from build123d import *

# Parameters (mm, degrees)
SKETCH1_R           = 100
SKETCH1_R_2         = 1.75
BOSS_EXTRUDE1_DEPTH = 2
BOSS_EXTRUDE2_DEPTH = 2


with BuildPart() as part:
    # Sketch1 → Boss-Extrude1 (new body)
    with BuildSketch(Plane.XY):
        Circle(SKETCH1_R)
        Circle(SKETCH1_R_2, mode=Mode.SUBTRACT)
    extrude(amount=BOSS_EXTRUDE1_DEPTH)

    # Sketch2 → Boss-Extrude2 (add)
    with BuildSketch(Plane.XY.offset(2)):
        Polygon((-1.25, -86), (1.25, -86), (3.25, -84), (-3.25, -84), align=None)
        Polygon((42.41156908, -80.578044827), (39.374382907, -74.271262752), (38.440212649, -76.940967966), (40.175747605, -80.544843437), align=None)
        Polygon((78.645827138, -58.561048264), (73.173006761, -54.196619651), (72.707858639, -56.383772418), (75.835184569, -58.877731625), align=None)
        Polygon((93.314928402, -22.58066955), (94.819742358, -24.975567242), (96.266128429, -18.638535813), (93.871230737, -20.14334977), align=None)
        Polygon((89.971519088, 19.253266034), (89.441633044, 17.080889275), (96.266128429, 18.638535813), (93.871230737, 20.14334977), align=None)
        Polygon((68.016869745, 52.642833607), (67.700186383, 49.832191038), (73.173006761, 54.196619651), (71.144195674, 55.136792814), align=None)
        Polygon((40.175747605, 80.544843437), (42.41156908, 80.578044827), (41.043515084, 82.346781173), align=None)
        Polygon((37.923325436, 81.629552785), (40.175747605, 80.544843437), (41.043515084, 82.346781173), (38.791092914, 83.431490521), align=None)
        Polygon((38.791092914, 83.431490521), (36.555271439, 83.398289131), (37.923325436, 81.629552785), align=None)
        Polygon((1.25, 86), (-1.25, 86), (-3.25, 84), (3.25, 84), align=None)
        Polygon((-42.41156908, 80.578044827), (-39.374382907, 74.271262752), (-38.440212649, 76.940967966), (-40.175747605, 80.544843437), align=None)
        Polygon((-78.645827138, 58.561048264), (-73.173006761, 54.196619651), (-72.707858639, 56.383772418), (-75.835184569, 58.877731625), align=None)
        Polygon((-93.314928402, 22.58066955), (-94.819742358, 24.975567242), (-96.266128429, 18.638535813), (-93.871230737, 20.14334977), align=None)
        Polygon((-89.971519088, -19.253266034), (-89.441633044, -17.080889275), (-96.266128429, -18.638535813), (-93.871230737, -20.14334977), align=None)
        Polygon((-68.016869745, -52.642833607), (-67.700186383, -49.832191038), (-73.173006761, -54.196619651), (-71.144195674, -55.136792814), align=None)
        Polygon((-40.175747605, -80.544843437), (-42.41156908, -80.578044827), (-41.043515084, -82.346781173), align=None)
        Polygon((-37.923325436, -81.629552785), (-40.175747605, -80.544843437), (-41.043515084, -82.346781173), (-38.791092914, -83.431490521), align=None)
        Polygon((-38.791092914, -83.431490521), (-36.555271439, -83.398289131), (-37.923325436, -81.629552785), align=None)
    extrude(amount=BOSS_EXTRUDE2_DEPTH)


solid = part.part
Can you work these out from the model? Positions are in its coordinate system, mm. A direction names the side the tool comes from. Coordinates: 2 decimals unless noted, no trailing zeros. Loops run counter-clockwise (first coordinate to the right, second up) from the corner with the lowest first, then second, coordinate; pieces in that order, holes last. Notation, with made-up numbers: M 46.25,86 L 91.25,86 A24 ccw 91.25,124 Z; hole C 51.25,68 d9. An arc over 180 degrees is marked long. Return JSON: item names as keys, results as strings. Group by question number.
Item 1: I'm going to push flat-ended pins straight in: pin 1 Ø1 at (y, z) = (-51, 1.5) entering from -X; pin 2 Ø2 at (x, y) = (-24, -74.5) entering from -Z; pin 3 Ø1.6 at (x, z) = (1.5, 3) entering from +Y; pin 4 Ø1.6 at (x, z) = (-1, 3.5) entering from -Y. Where does each tip first touch, or does it pass through?
Item 2: If I drill on L1, parallel to Y at x = 0, z = 1.45; L2, parallel to Z at x = 38.5, y = 15.5; L3, parallel to X at y = 80.5, z = 3.35, over which ranges is the centre line in solid material (lowest first)? Write a range as from..to.
Item 3: On a 3-axis mill with a long thin cutter (end or side, diameter ignored), from which of +Z, -Z, +X, -X, +Y, -Y can I reach the whole of each face in a straight line? I mean faces 1 (the flat face through (-75.95, 56.41, 2.99)), 2 (the flat face through (70, 53, 4)), 3 (the flat face through (75.95, -56.41, 2.99)). Say none if no direction works.
Item 4: Imagine slicing it at A-A (z = 2.7). Give the number of separate pieces and of enclosed holes in the cut face, and give its area (3 significant figures).
Item 5: Imagine slicing it at B-B (x = 61). Please give me the cut outline in (y, z), and give its area (3 significant figures).
Item 6: Imagine slicing it at C-C (y = 31). Please give me the cut outline in (x, z).
Verdict:
{
 "1": {"pin 1": "stops at x = -86.31", "pin 2": "stops at z = 0", "pin 3": "stops at y = 86", "pin 4": "stops at y = -86"},
 "2": {"L1": "y = -100..-1.75, 1.75..100", "L2": "z = 0..2", "L3": "x = -42.37..-40.15"},
 "3": {"face 1": "+Z, -X, -Y", "face 2": "+Z, +X, -X, +Y, -Y", "face 3": "+Z, +X, +Y"},
 "4": {"separate pieces": "14", "enclosed holes": "0", "area": "142 mm^2"},
 "5": {"outline": "M -79.24,0 L 79.24,0 L 79.24,2 L -79.24,2 Z", "area": "317 mm^2"},
 "6": {"outline": "M -95.07,0 L 95.07,0 L 95.07,2 L -95.07,2 Z"}
}
